```python
from build123d import *

# Parameters (mm, degrees)
BOSS_EXTRUDE1_DEPTH      = 105
BOSS_EXTRUDE1_DEPTH_BACK = 10
SKETCH1_R                = 157.5
SKETCH1_R_2              = 125
SKETCH3_R                = 4
CUT_EXTRUDE2_DEPTH       = 251.674091202
CIRPATTERN2_COUNT        = 12


with BuildPart() as part:
    # Sketch1 → Boss-Extrude1 (new, two sides: drawn at the far end of the back side and taken through both)
    with BuildSketch(Plane(origin=(0, 0, 0), x_dir=(1, 0, 0), z_dir=(0, 1, 0)).offset(-BOSS_EXTRUDE1_DEPTH_BACK)):
        with Locations(Location((0, 0, 0), (0, 0, 270))):
            Circle(SKETCH1_R)
        with Locations(Location((0, 0, 0), (0, 0, 270))):
            Circle(SKETCH1_R_2, mode=Mode.SUBTRACT)
    extrude(amount=BOSS_EXTRUDE1_DEPTH + BOSS_EXTRUDE1_DEPTH_BACK)

    # Sketch3 → Cut-Extrude2 (cut, through all)
    with BuildSketch(Plane(origin=(0, -10, 0), x_dir=(-1, 0, 0), z_dir=(0, -1, 0))):
        with Locations(Location((-15, 141.25, 0), (0, 0, 90))):
            Circle(SKETCH3_R)
        with Locations(Location((15, 141.25, 0), (0, 0, 270))):
            Circle(SKETCH3_R)
    cut_extrude2 = extrude(amount=-CUT_EXTRUDE2_DEPTH, mode=Mode.SUBTRACT)

    # CirPattern2: Cut-Extrude2 ×12 about axis
    cirpattern2_axis = Axis((0, 0, 0), (0, 1, 0))
    for i in range(1, CIRPATTERN2_COUNT):
        add(cut_extrude2.rotate(cirpattern2_axis, i * 360 / CIRPATTERN2_COUNT), mode=Mode.SUBTRACT)


solid = part.part
```
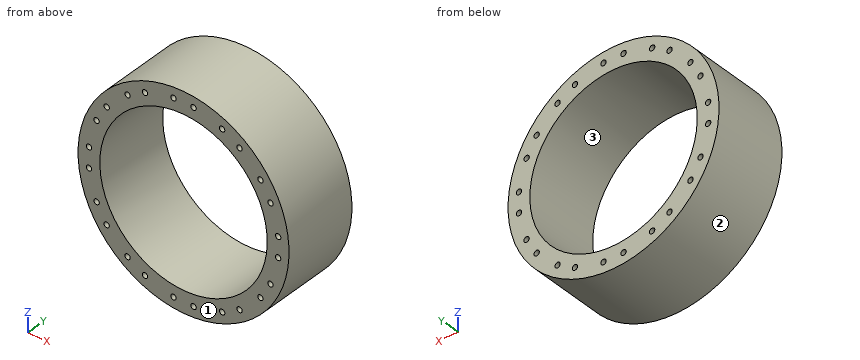
Can you work these out from the model? Positions are in its coordinate system, mm. Face numbers are marked on the shaded views. Coordinates: 2 decimals unless noted, no trailing zeros. Order: outer loops, then holes, each group sorted by start corner. A loop starts at its lowest first (then second) coordinate and runs counter-clockwise, first axis right, second up.
1. If we section it at D-D (x = -141.25): Please give me the cut outline in (y, z), then the cut area to 3 significant figures.
2. I need wall thicknesses on line 1 (Z direction, x = 57.5, y = 26.5); line 2 (X direction, y = 20, z = 15.5); line 3 (Z direction, x = 139.5, y = 90.5). Which ranges of each line are inside material? Lowest first, please.
3. If we section it at C-C (z = -141.25): Please give me the cut outline in (x, y).
4. If we section it at A-A (x = 0): Please give me the cut outline in (y, z), then the cut area to 4 significant figures.
5. Thinking about a two-plate mould opening in X: for the marked faces 1, 2 and 3, which applies, +X half, -X half, draft (parallel to the pull), parting line (faces both ways), or undercut?
6. If we section it at B-B (z = 0): Please give me the cut outline in (x, y).
7. I'm going to push flat-ended pins straight in: pin 1 (2 mm diameter, centred on y = 77, z = 9, fed in from -X); pin 2 (1.5 mm diameter, centred on y = 66.5, z = 114, fed in from -X); pin 3 (1 mm diameter, centred on y = 47.5, z = -110.5, fed in from -X). Where does each tip first touch, or does it pass through?
Entries:
1. outline: (-10, -69.68) - (105, -69.68) - (105, -19) - (-10, -19) - close; (-10, -11) - (105, -11) - (105, 11) - (-10, 11) - close; (-10, 19) - (105, 19) - (105, 69.68) - (-10, 69.68) - close
1. area: 14,200 mm2
2. line 1: z = -146.63 to -133.82, -125.83 to -110.99, 110.99 to 125.83, 133.82 to 146.63
2. line 2: x = -156.74 to -145.22, -137.28 to -124.04, 124.04 to 137.28, 145.22 to 156.74
2. line 3: z = -73.12 to -18.6, -11.4 to 11.4, 18.6 to 73.12
3. outline: (-69.68, -10) - (-19, -10) - (-19, 105) - (-69.68, 105) - close; (-11, -10) - (11, -10) - (11, 105) - (-11, 105) - close; (19, -10) - (69.68, -10) - (69.68, 105) - (19, 105) - close
4. outline: (-10, -157.5) - (105, -157.5) - (105, -125) - (-10, -125) - close; (-10, 125) - (105, 125) - (105, 157.5) - (-10, 157.5) - close
4. area: 7,475 mm2
5. face 1: draft
5. face 2: parting line
5. face 3: undercut
6. outline: (-157.5, -10) - (-125, -10) - (-125, 105) - (-157.5, 105) - close; (125, -10) - (157.5, -10) - (157.5, 105) - (125, 105) - close
7. pin 1: stops at x = -157.3
7. pin 2: stops at x = -109.46
7. pin 3: stops at x = -112.72
